Input: part model. Units: mm. Frame: model coordinates. Face numbers are marked on the shaded views. A direction names the side the tool comes from. Round coordinates to 2 decimals unless told otherwise and drop trailing zeros. Loops run counter-clockwise (first coordinate to the right, second up) from the corner with the lowest first, then second, coordinate; pieces in that order, holes last.
(1) Access query for the marked faces 1, 2, 3, 4 and 5. Directions: +Z, -Z, +X, -X, +Y, -Y. A direction counts if a zero-diameter tool reaches every point of the face in a straight line with its end or side. Return the directions, or none.
(2) Cut plane D-D, the plane x = -15. Output: boundary loops of the cut face in (y, z).
(3) Line query: line 1 (Y direction, x = 0, z = -3.45); line 2 (Y direction, x = 0, z = 7); line 3 (Z direction, x = 3, y = 24). Output: solid intervals per line, ascending.
(4) Cut plane C-C, the plane z = 9. Output: boundary loops of the cut face in (x, y), and give its area (3 significant figures).
(5) First-contact query: pin 1 Ø5 at (x, y) = (-1.5, -23.5) entering from +Z; pin 2 Ø12 at (x, y) = (13, 9) entering from +Z; pin 3 Ø9 at (x, y) = (0, 0) entering from +Z; pin 4 Ø8.5 at (x, y) = (-0.5, 2) entering from -Z. Flat tips, straight axial feed; report the tip coordinate or a pass-through.
(6) Cut plane B-B, the plane y = 0. Output: boundary loops of the cut face in (x, z), and give its area (3 significant figures).
(7) Draft query along X for the marked faces 6, 7 and 8. Return one class per face: released by +X, released by -X, zero draft, split by the parting line, or undercut.
from build123d import *

# Parameters (mm, degrees)
SKETCH_1_R          = 17
EXTRUDE_1_DEPTH     = 6
SKETCH_2_R          = 7
EXTRUDE_2_DEPTH     = 6
SKETCH_3_R          = 18
EXTRUDE_3_DEPTH     = 5
EXTRUDE_START       = -5
EXTRUDE_6_DEPTH     = 5
CUT_EXTRUDE_1_DEPTH = 8
SKETCH_6_R          = 3.275
EXTRUDE_5_DEPTH     = 4.4
SKETCH_9_R          = 5
CUT_EXTRUDE_3_DEPTH = 37.608729958
SKETCH_10_R         = 13.6
SKETCH_10_R_2       = 8.6
CUT_EXTRUDE_4_DEPTH = 3
SKETCH_11_R         = 8.6
CUT_EXTRUDE_5_DEPTH = 2.8


with BuildPart() as part:
    # 스케치1 → 보스-돌출1 (new body)
    with BuildSketch(Plane.XY):
        Circle(SKETCH_1_R)
    extrude(amount=EXTRUDE_1_DEPTH)

    # 스케치2 → 보스-돌출2 (add)
    with BuildSketch(Plane.XY.offset(6)):
        Circle(SKETCH_2_R)
    extrude(amount=EXTRUDE_2_DEPTH)

    # 스케치3 → 보스-돌출3 (add)
    with BuildSketch(Plane(origin=(0, 0, 0), x_dir=(-1, 0, 0), z_dir=(0, 0, -1))):
        Circle(SKETCH_3_R)
    extrude(amount=EXTRUDE_3_DEPTH)

    # 스케치8 → 보스-돌출6 (add)
    with BuildSketch(Plane(origin=(0, 0, -5), x_dir=(-1, 0, 0), z_dir=(0, 0, -1)).offset(EXTRUDE_START)):
        with BuildLine():
            Line((-10, 14.966629547), (-10, 26.966629547))
            Line((-10, 26.966629547), (10, 26.966629547))
            Line((10, 26.966629547), (10, 14.966629547))
            ThreePointArc((10, 14.966629547), (0, 18), (-10, 14.966629547))
        make_face()
    extrude_6 = extrude(amount=EXTRUDE_6_DEPTH)

    # 스케치5 → 컷-돌출1 (cut)
    with BuildSketch(Plane.XY):
        Polygon((-10, 27), (-10, 15), (-4, 27), align=None)
        Polygon((4, 27), (10, 27), (10, 15), align=None)
    cut_extrude_1 = extrude(amount=-CUT_EXTRUDE_1_DEPTH, mode=Mode.SUBTRACT)

    # 스케치6 → 보스-돌출5 (add)
    with BuildSketch(Plane.XY):
        with Locations(Location((0, 21.966629547, 0), (0, 0, 180))):
            Circle(SKETCH_6_R)
    extrude_5 = extrude(amount=EXTRUDE_5_DEPTH)

    # 대칭 복사6: 보스-돌출6, 컷-돌출1, 보스-돌출5 across plane
    add(extrude_6.mirror(Plane.ZX))
    add(cut_extrude_1.mirror(Plane.ZX), mode=Mode.SUBTRACT)
    add(extrude_5.mirror(Plane.ZX))

    # 스케치9 → 컷-돌출3 (cut, through all)
    with BuildSketch(Plane.XY.offset(12)):
        Circle(SKETCH_9_R)
    extrude(amount=-CUT_EXTRUDE_3_DEPTH, mode=Mode.SUBTRACT)

    # 스케치10 → 컷-돌출4 (cut)
    with BuildSketch(Plane(origin=(0, 0, -5), x_dir=(-1, 0, 0), z_dir=(0, 0, -1))):
        Circle(SKETCH_10_R)
        Circle(SKETCH_10_R_2, mode=Mode.SUBTRACT)
    extrude(amount=-CUT_EXTRUDE_4_DEPTH, mode=Mode.SUBTRACT)

    # 스케치11 → 컷-돌출5 (cut)
    with BuildSketch(Plane(origin=(0, 0, -5), x_dir=(-1, 0, 0), z_dir=(0, 0, -1))):
        Circle(SKETCH_11_R)
    extrude(amount=-CUT_EXTRUDE_5_DEPTH, mode=Mode.SUBTRACT)


solid = part.part
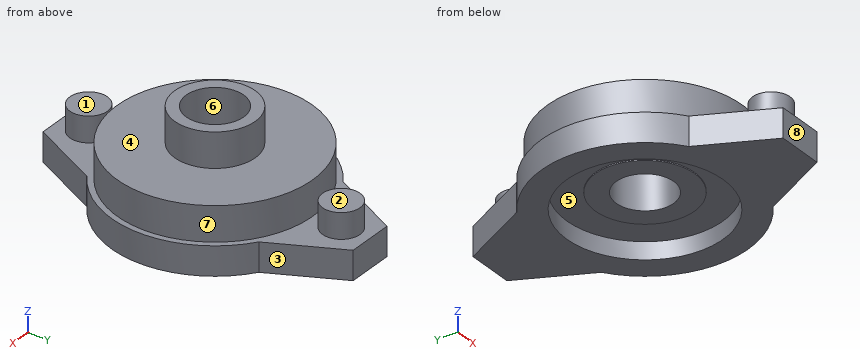
Reported:
1. face 1: +Z, +X, -X, -Y
1. face 2: +Z, +X, -X, +Y
1. face 3: +Z, -Z, +X, +Y
1. face 4: +Z
1. face 5: -Z
2. outline: (-9.95, -5) - (9.95, -5) - (9.95, 0) - (8, 0) - (8, 6) - (-8, 6) - (-8, 0) - (-9.95, 0) - close
3. line 1: y = -26.97 to -13.6, 13.6 to 26.97
3. line 2: y = -7 to -5, 5 to 7
3. line 3: z = -5 to 0
4. outline: circle Ø14 at (0, 0); hole circle Ø10 at (0, 0)
4. area: 75.4 mm2
5. pin 1: stops at z = 4.4
5. pin 2: stops at z = 6
5. pin 3: passes through
5. pin 4: stops at z = -2.2
6. outline: (-18, -5) - (-13.6, -5) - (-13.6, -2) - (-8.6, -2) - (-8.6, -2.2) - (-5, -2.2) - (-5, 12) - (-7, 12) - (-7, 6) - (-17, 6) - (-17, 0) - (-18, 0) - close; (5, -2.2) - (8.6, -2.2) - (8.6, -2) - (13.6, -2) - (13.6, -5) - (18, -5) - (18, 0) - (17, 0) - (17, 6) - (7, 6) - (7, 12) - (5, 12) - close
6. area: 248 mm2
7. face 6: undercut
7. face 7: split by the parting line
7. face 8: zero draft
